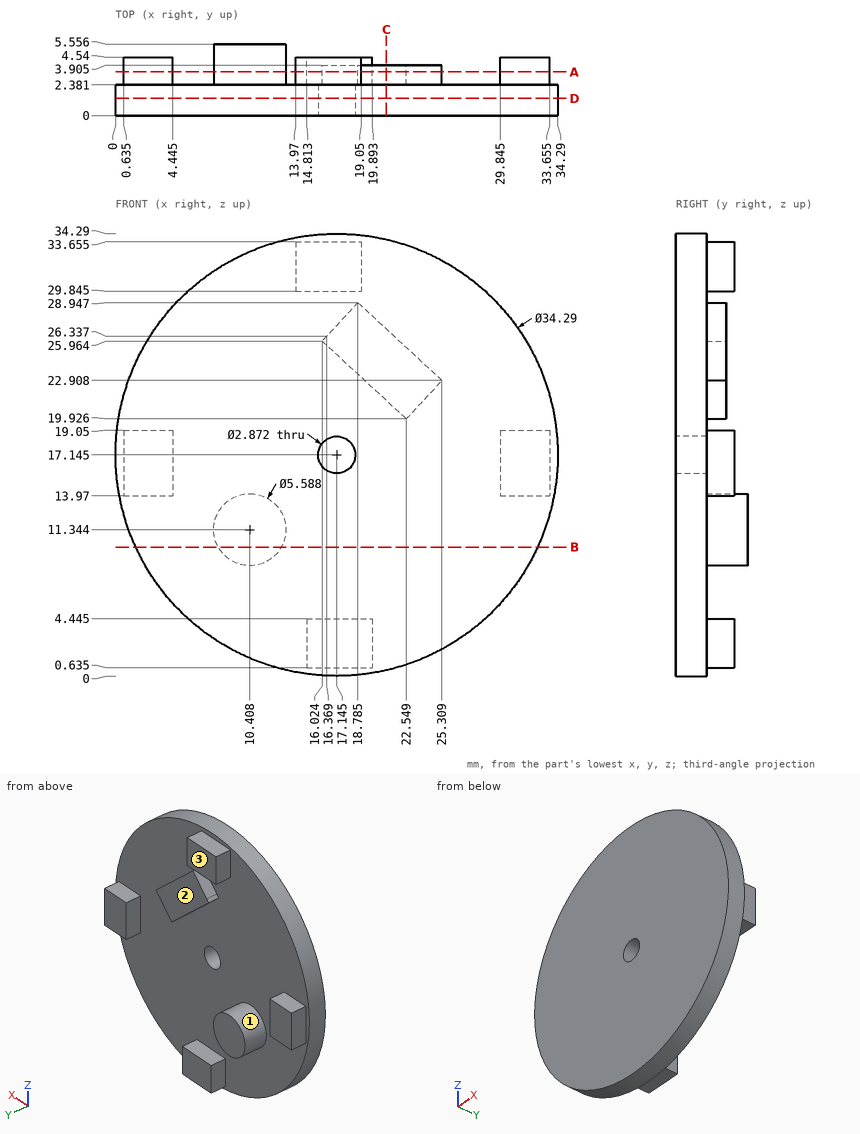
Answer from the drawing. Dimensions are ordinates in mm from the lowest x, y and z of the part. A direction names the side the tool comes from. Give positions to 0.01 mm unless a question says otherwise; leave off trailing zeros. Order: outer loops, then holes, each group sorted by start corner. A loop starts at its lowest first (then second) coordinate and runs counter-clockwise, first axis right, second up. Notation, with made-up numbers: (18.25, 58.25) -> (66.25, 58.25) arc R21 ccw to (66.25, 65.25) -> close; hole circle Ø2 at (-2.5, 65.25). An arc over 180 degrees is marked (long way). One line per item, written item: value.
Item 1: Straight lines are drawn through the part: probe 1 along Y at (x, z) = (15.5, 4); probe 2 along Y at (x, z) = (23, 3); probe 3 along X at (y, z) = (4.35, 32). For each, find the intervals that lie inside material, in ascending order.
Answer sheet:
probe 1: 0 to 4.54
probe 2: 0 to 2.38
probe 3: 13.97 to 19.05
Item 2: Find section A-A, the plane y = 3.4. State how many separate pieces and enclosed holes the cut face has, plus the area to 3 significant figures.
Answer sheet:
separate pieces: 6
enclosed holes: 0
area: 138 mm²
Item 3: Flat-ended cylindrical pins translate along their axes: P1, Ø8, axis at x = 16, z = 4.5, coming from the -Y side; P2, Ø1, axis at y = 1.5, z = 7, coming from the +X side; P3, Ø1.7, axis at y = 4, z = 31.5, coming from the +X side; P4, Ø0.6, axis at x = 18.5, y = 3, coming from the +Z side (1 decimal). Find the tip coordinate at first contact, or state that the pin passes through.
Answer sheet:
P1: y = 0
P2: x = 31.32
P3: x = 19.05
P4: z = 33.7
Item 4: Find section D-D, the plane y = 1.35. Give the vertices of the cut face in (x, z) (1 decimal).
Answer sheet:
outline: circle Ø34.3 at (17.1, 17.1); hole circle Ø2.9 at (17.1, 17.1)
Item 5: Find section C-C, the plane x = 21. Give the vertices of the cut face in (y, z) (1 decimal).
Answer sheet:
outline: (0, 0.4) -> (2.4, 0.4) -> (2.4, 21.4) -> (3.9, 21.4) -> (3.9, 26.9) -> (2.4, 26.9) -> (2.4, 33.9) -> (0, 33.9) -> close
Item 6: A tool of negligible diameter and unlimited length cuts with its end or side. For the marked faces 1, 2 and 3, from which of +Z, -Z, +X, -X, +Y, -Y can it reach the whole face along a straight path? Write none if from no direction.
Answer sheet:
face 1: +Y
face 2: +X, -X, +Y
face 3: +Z, -Z, +X, -X, +Y
Item 7: Find section B-B, the plane z = 10. Give the vertices of the cut face in (x, y).
Answer sheet:
outline: (1.56, 0) -> (32.73, 0) -> (32.73, 2.38) -> (12.86, 2.38) -> (12.86, 5.56) -> (7.96, 5.56) -> (7.96, 2.38) -> (1.56, 2.38) -> close
